Geometry: see drawing. Coordinates: mm, zero at the bounding-box minimum. A direction names the side the tool comes from. Coordinates: 2 decimals unless noted, no trailing zeros. Write each loop counter-clockwise with the first axis right and the second up, starting at its lowest first coordinate (ties: lowest second). Pieces come first, ordered by that corner, then holes. Notation, with made-up numbers: (-17, 65) - (-1, 65) arc R20 ccw to (-1, 90) - close; hole circle Ø7 at (87.25, 78.5). An arc over 180 degrees is marked (long way). One line per question, with ' | ' between items. Start each with the question number.
1) Section query A-A on x = 88.1. Return loops of the section in (y, z) (1 decimal).
2) Section query B-B on x = 154. Give the number of separate pieces and of enclosed holes in the cut face, and give its area (3 significant figures).
3) Draft query along X for the marked faces 3, 4 and 5. Return one class per face: released by +X, released by -X, zero draft, split by the parting line, or undercut.
4) Section query C-C on y = 29. Return loops of the section in (x, z) (1 decimal).
5) Line query: line 1 (X direction, y = 41, z = 23.75) (1 decimal); line 2 (X direction, y = 59, z = 9.75); line 3 (X direction, y = 47, z = 15) (1 decimal). Output: solid intervals per line, ascending.
6) First-contact query: P1, Ø10, axis at x = 81, y = 48.5, coming from the +Z side. Flat tip, straight axial feed; report the tip coordinate or a pass-through.
7) Reachability of the marked faces 1 and 2 from +Z, -Z, +X, -X, +Y, -Y: full face, straight path, thin tool, end or side. Return the list, or none.
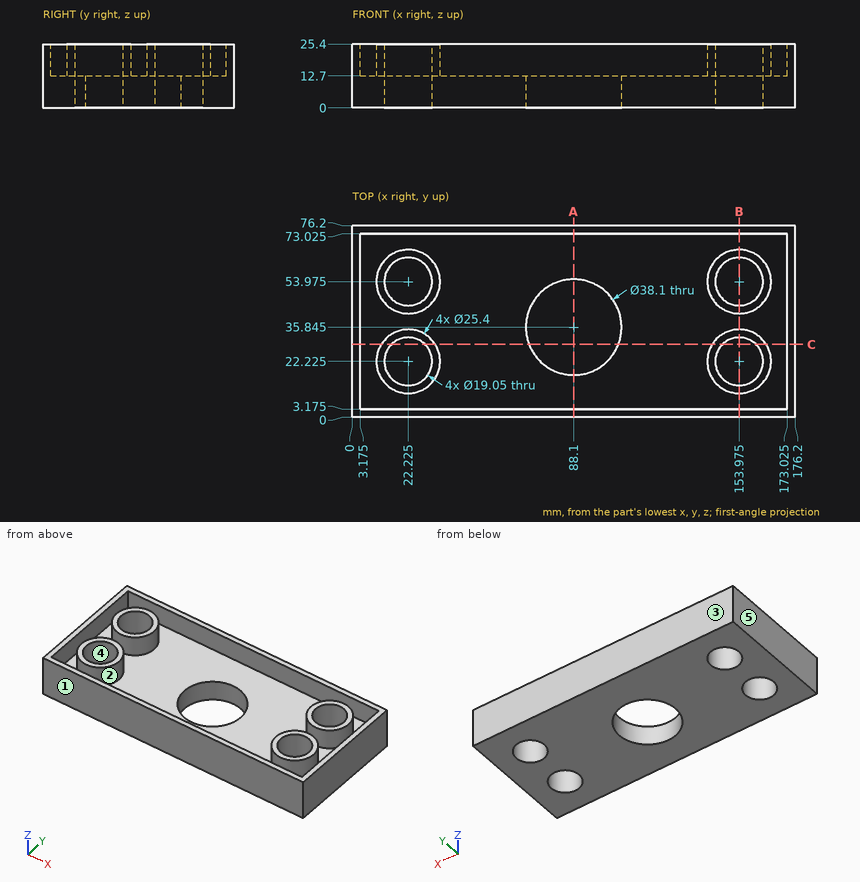
Answer key:
1) outline: (0, 0) - (16.8, 0) - (16.8, 12.7) - (3.2, 12.7) - (3.2, 25.4) - (0, 25.4) - close; (54.9, 0) - (76.2, 0) - (76.2, 25.4) - (73, 25.4) - (73, 12.7) - (54.9, 12.7) - close
2) separate pieces: 3 | enclosed holes: 0 | area: 726 mm²
3) face 3: zero draft | face 4: undercut | face 5: released by -X
4) outline: (0, 0) - (15.5, 0) - (15.5, 25.4) - (11.5, 25.4) - (11.5, 12.7) - (3.2, 12.7) - (3.2, 25.4) - (0, 25.4) - close; (28.9, 0) - (70.3, 0) - (70.3, 12.7) - (33, 12.7) - (33, 25.4) - (28.9, 25.4) - close; (105.9, 0) - (147.3, 0) - (147.3, 25.4) - (143.2, 25.4) - (143.2, 12.7) - (105.9, 12.7) - close; (160.7, 0) - (176.2, 0) - (176.2, 25.4) - (173, 25.4) - (173, 12.7) - (164.7, 12.7) - (164.7, 25.4) - (160.7, 25.4) - close
5) line 1: 0 to 3.2, 173 to 176.2 | line 2: 0 to 14.13, 30.32 to 145.88, 162.07 to 176.2 | line 3: 0 to 3.2, 11.6 to 15.7, 28.7 to 32.8, 143.4 to 147.5, 160.5 to 164.6, 173 to 176.2
6) P1: z = 12.7
7) face 1: +Z, -Z, +X, -X, -Y | face 2: +Z
